Design review of the part built by this model. Coordinates are the model's own, in mm. A direction names the side the tool comes from. Coordinates: 2 decimals unless noted, no trailing zeros. Order: outer loops, then holes, each group sorted by start corner. A loop starts at its lowest first (then second) coordinate and runs counter-clockwise, first axis right, second up. Notation, with made-up numbers: (-1, -39.5) -> (40, -39.5) arc R19 ccw to (40, -9.5) -> close; hole circle Ø9 at (44.5, -3.75). An arc over 180 degrees is marked (long way). Write item = value, one per line.
```python
from build123d import *

# Parameters (mm, degrees)
SKETCH1_W           = 393.7
SKETCH1_H           = 100.9392952
BOSS_EXTRUDE1_DEPTH = 6.35
SKETCH2_W           = 393.4968
SKETCH2_H           = 100.7360952
BOSS_EXTRUDE2_DEPTH = 6.35


with BuildPart() as part:
    # Sketch1 → Boss-Extrude1 (new body)
    with BuildSketch(Plane(origin=(0, 0, 0), x_dir=(1, 0, 0), z_dir=(0, 1, 0))):
        Polygon((196.85, 58.683525), (203.2, 58.683525), (203.2, -58.683525), (196.85, -58.683525), (196.85, -56.8196476), (-196.85, -56.8196476), (-196.85, -58.683525), (-203.2, -58.683525), (-203.2, 58.683525), (-196.85, 58.683525), (-196.85, 56.8196476), (196.85, 56.8196476), align=None)
        Rectangle(SKETCH1_W, SKETCH1_H, mode=Mode.SUBTRACT)
    extrude(amount=BOSS_EXTRUDE1_DEPTH)

    # Sketch2 → Boss-Extrude2 (add)
    with BuildSketch(Plane(origin=(0, 6.35, 0), x_dir=(1, 0, 0), z_dir=(0, 1, 0))):
        Polygon((196.7484, -58.785125), (203.3016, -58.785125), (203.3016, 58.785125), (196.7484, 58.785125), (196.7484, 56.9212476), (-196.7484, 56.9212476), (-196.7484, 58.785125), (-203.3016, 58.785125), (-203.3016, -58.785125), (-196.7484, -58.785125), (-196.7484, -56.9212476), (196.7484, -56.9212476), align=None)
        Rectangle(SKETCH2_W, SKETCH2_H, mode=Mode.SUBTRACT)
    extrude(amount=-BOSS_EXTRUDE2_DEPTH)


solid = part.part
```
(1) For faces 4 (the flat face through (3, 3, -56.921)), 5 (the flat face through (-3, 3, 56.921)), 6 (the flat face through (-200, 3, -58.785)), 7 (the flat face through (-196.748, 3, 1)), list the 3-axis set-ups (+Z, -Z, +X, -X, +Y, -Y) from which the entire face can be reached by the end or side of a thin tool; tool diameter is ignored.
Report:
face_4 = -Z, +Y, -Y
face_5 = +Z, +Y, -Y
face_6 = -Z, +X, -X, +Y, -Y
face_7 = +Y, -Y
(2) We need section B-B (z = -15.5). Write out the cut boundary in (x, y), and give its area (3 significant figures).
Report:
outline = (-203.3, 0) -> (-196.75, 0) -> (-196.75, 6.35) -> (-203.3, 6.35) -> close; (196.75, 0) -> (203.3, 0) -> (203.3, 6.35) -> (196.75, 6.35) -> close
area = 83.2 mm²
(3) We need section A-A (x = -83.5). Write out the cut boundary in (y, z).
Report:
outline = (0, -56.92) -> (6.35, -56.92) -> (6.35, -50.37) -> (0, -50.37) -> close; (0, 50.37) -> (6.35, 50.37) -> (6.35, 56.92) -> (0, 56.92) -> close
(4) Insertion check: pin 1 (3 mm diameter, centred on x = -13, y = 2, fed in from -Z); pin 2 (1.9 mm diameter, centred on x = -94.5, y = 3.5, fed in from +Z). Each pin has a flat end and moves straight along its axis. Give the tip position at first contact, or say it passes through.
Report:
pin_1 = -56.92
pin_2 = 56.92
(5) For L1, parallel to Z at x = -68, y = 0.5; L2, parallel to X at y = 2.25, z = -8, list the stretches that pass through material, from the lowest coordinate up.
Report:
L1 = -56.92 to -50.37, 50.37 to 56.92
L2 = -203.3 to -196.75, 196.75 to 203.3
(6) The part is to be moulded in two halves that separate along Z. For faces 1 (the flat face through (203.302, 3, 1)), 2 (the flat face through (-3, 3, 50.368)), 3 (the flat face through (200, 3, 58.785)), say which applies: released by +Z, released by -Z, zero draft, split by the parting line, or undercut.
Report:
face_1 = zero draft
face_2 = undercut
face_3 = released by +Z
(7) We need section C-C (y = 3.75). Write out the cut boundary in (x, z).
Report:
outline = (-203.3, -58.79) -> (-196.75, -58.79) -> (-196.75, -56.92) -> (196.75, -56.92) -> (196.75, -58.79) -> (203.3, -58.79) -> (203.3, 58.79) -> (196.75, 58.79) -> (196.75, 56.92) -> (-196.75, 56.92) -> (-196.75, 58.79) -> (-203.3, 58.79) -> close; hole (-196.75, -50.37) -> (196.75, -50.37) -> (196.75, 50.37) -> (-196.75, 50.37) -> close
